Design review of the part built by this model. Coordinates are the model's own, in mm. A direction names the side the tool comes from. Give positions to 0.01 mm unless a question says otherwise; leave off trailing zeros. Order: outer loops, then holes, each group sorted by start corner. A loop starts at its lowest first (then second) coordinate and runs counter-clockwise, first axis right, second up. Notation, with made-up numbers: (-24, -34) -> (-6, -34) arc R15 cw to (-6, -17) -> close; hole circle Ø7 at (3, 52). An arc over 180 degrees is marked (long way). One line per item, written item: value. Start each with the question number.
1) Consider section B-B (z = 28). State the section outline as (x, y) points.
2) Consider section A-A (y = 101.5). State the section outline as (x, z) points.
3) Tool access review of faces 4 (the face through (-14.616, -3, 26)), 5 (the face through (16.42, -3.19, 45.49)), 6 (the face through (27, -3, 12.27)): name each direction out of +Z, -Z, +X, -X, +Y, -Y from which nothing blocks a thin tool from reaching the whole face with its end or side.
4) For pin 1 (9 mm diameter, centred on y = 33, z = 25, fed in from -X); pin 2 (1 mm diameter, centred on x = -26, y = 162.5, fed in from +Z); pin 3 (8 mm diameter, centred on x = -2.5, y = -14, fed in from +Z); pin 4 (12 mm diameter, centred on x = -29, z = 22.5, fed in from +Y), all flat-tipped, find the tip position at first contact; note any pin that passes through.
5) Wall thickness on line 1 along X through (y, z) = (58, 29); line 2 along Z through (x, y) = (34, 103.5); line 3 along Z through (x, y) = (18.5, -6): over which ranges is each line inside the solid? List them lowest first. Write a range as from..to.
6) The part is to be moulded in two halves that separate along Z. For faces 1 (the face through (1, -227.892, 19)), 2 (the face through (-26, -3, 12.27)), 3 (the face through (0.066, 3.19, 45.438)), say which applies: released by +Z, released by -Z, zero draft, split by the parting line, or undercut.
from build123d import *

# Parameters (mm, degrees)
F1_DEPTH    = 227.8918027878
F3_D        = 12.7
F4_T1_DEPTH = 455.7836055756
F4_T3_DEPTH = 473.2454690546
F4_T5_DEPTH = 481.1836055756
F4_T7_DEPTH = 475.2289422773


# Not quite as in the source:
# - a fillet or chamfer that OpenCascade refuses, or shapes differently, is made with other operations: its cross-section is extruded or revolved along the edge and cut away or added


with BuildPart() as f1:
    # F0 (on Front) → F1 (new body, symmetric)
    with BuildSketch(Plane.XZ):
        Polygon((-38.2542312145, 0), (0, 0), (38.2542312145, 0), (38.2542312145, 12.2701972723), (14.6159976721, 12.2701972723), (14.6159976721, 35.1866483688), (26.3448953629, 35.1866483688), (26.3448953629, 41.6826456785), (0, 51.7875403166), (-26.3448953629, 41.6826456785), (-26.3448953629, 35.1866483688), (-14.6159976721, 35.1866483688), (-14.6159976721, 12.2701972723), (-38.2542312145, 12.2701972723), align=None)
    extrude(amount=F1_DEPTH, both=True)

    # F3 (through all)
    with Locations(Plane.XZ.offset(227.8918027878)):
        with Locations((0, 51.7875403166)):
            Hole(F3_D / 2)

    # F4: fillet of radius 5.08 on 12 edges, made by hand

    # F4_s2 → F4_t1 (join)
    with BuildSketch(Plane.XZ.offset(-227.8918027878)):
        with BuildLine():
            ThreePointArc((-19.6959976721, 12.2701972723), (-16.1038952237, 13.7580948239), (-14.6159976721, 17.3501972723))
            Line((-14.6159976721, 17.3501972723), (-14.6159976721, 12.2701972723))
            Line((-14.6159976721, 12.2701972723), (-19.6959976721, 12.2701972723))
        make_face()
        with BuildLine():
            ThreePointArc((14.6159976721, 17.3501972723), (16.1038952237, 13.7580948239), (19.6959976721, 12.2701972723))
            Line((19.6959976721, 12.2701972723), (14.6159976721, 12.2701972723))
            Line((14.6159976721, 12.2701972723), (14.6159976721, 17.3501972723))
        make_face()
    extrude(amount=F4_T1_DEPTH)

    # F4_s4 → F4_t3 (cut)
    with BuildSketch(Plane.XZ.offset(-236.6227345273)):
        with BuildLine():
            ThreePointArc((23.0841549326, 42.9333410423), (25.4510773115, 41.0681681672), (26.3448953629, 38.1902729827))
            Line((26.3448953629, 38.1902729827), (26.3448953629, 41.6826456785))
            Line((26.3448953629, 41.6826456785), (23.0841549326, 42.9333410423))
        make_face()
        with BuildLine():
            ThreePointArc((-26.3448953629, 38.1902729827), (-25.4510773115, 41.0681681672), (-23.0841549326, 42.9333410423))
            Line((-23.0841549326, 42.9333410423), (-26.3448953629, 41.6826456785))
            Line((-26.3448953629, 41.6826456785), (-26.3448953629, 38.1902729827))
        make_face()
    extrude(amount=F4_T3_DEPTH, mode=Mode.SUBTRACT)

    # F4_s6 → F4_t5 (cut)
    with BuildSketch(Plane.XZ.offset(-240.5918027878)):
        with BuildLine():
            ThreePointArc((26.3448953629, 40.2666483688), (24.8569978113, 36.6745459204), (21.2648953629, 35.1866483688))
            Line((21.2648953629, 35.1866483688), (26.3448953629, 35.1866483688))
            Line((26.3448953629, 35.1866483688), (26.3448953629, 40.2666483688))
        make_face()
        with BuildLine():
            ThreePointArc((-21.2648953629, 35.1866483688), (-24.8569978113, 36.6745459204), (-26.3448953629, 40.2666483688))
            Line((-26.3448953629, 40.2666483688), (-26.3448953629, 35.1866483688))
            Line((-26.3448953629, 35.1866483688), (-21.2648953629, 35.1866483688))
        make_face()
        with BuildLine():
            ThreePointArc((38.2542312145, 7.1901972723), (36.766333663, 10.7822997207), (33.1742312145, 12.2701972723))
            Line((33.1742312145, 12.2701972723), (38.2542312145, 12.2701972723))
            Line((38.2542312145, 12.2701972723), (38.2542312145, 7.1901972723))
        make_face()
        with BuildLine():
            ThreePointArc((33.1742312145, 0), (36.766333663, 1.4878975516), (38.2542312145, 5.08))
            Line((38.2542312145, 5.08), (38.2542312145, 0))
            Line((38.2542312145, 0), (33.1742312145, 0))
        make_face()
        with BuildLine():
            ThreePointArc((-38.2542312145, 7.1901972723), (-36.766333663, 10.7822997207), (-33.1742312145, 12.2701972723))
            Line((-33.1742312145, 12.2701972723), (-38.2542312145, 12.2701972723))
            Line((-38.2542312145, 12.2701972723), (-38.2542312145, 7.1901972723))
        make_face()
        with BuildLine():
            ThreePointArc((-33.1742312145, 0), (-36.766333663, 1.4878975516), (-38.2542312145, 5.08))
            Line((-38.2542312145, 5.08), (-38.2542312145, 0))
            Line((-38.2542312145, 0), (-33.1742312145, 0))
        make_face()
    extrude(amount=F4_T5_DEPTH, mode=Mode.SUBTRACT)

    # F4_s8 → F4_t7 (cut)
    with BuildSketch(Plane.XZ.offset(-237.6144711386)):
        with BuildLine():
            ThreePointArc((-9.5599593035, 48.120705426), (-6.7869567139, 48.367304114), (-4.300388741, 47.1153720109))
            ThreePointArc((-4.300388741, 47.1153720109), (-5.2532816874, 48.2202540213), (-5.9288350745, 49.5134658544))
            Line((-5.9288350745, 49.5134658544), (-9.5599593035, 48.120705426))
        make_face()
        with BuildLine():
            ThreePointArc((4.300388741, 47.1153720109), (6.7869567139, 48.367304114), (9.5599593035, 48.120705426))
            Line((9.5599593035, 48.120705426), (5.9288350745, 49.5134658544))
            ThreePointArc((5.9288350745, 49.5134658544), (5.2532816874, 48.2202540213), (4.300388741, 47.1153720109))
        make_face()
    extrude(amount=F4_T7_DEPTH, mode=Mode.SUBTRACT)


solid = f1.part
Checked values:
1. outline: (-14.62, -227.89) -> (14.62, -227.89) -> (14.62, 227.89) -> (-14.62, 227.89) -> close
2. outline: (-38.25, 5.08) arc R5.08 ccw to (-33.17, 0) -> (33.17, 0) arc R5.08 ccw to (38.25, 5.08) -> (38.25, 7.19) arc R5.08 ccw to (33.17, 12.27) -> (19.7, 12.27) arc R5.08 cw to (14.62, 17.35) -> (14.62, 35.19) -> (21.26, 35.19) arc R5.08 ccw to (26.24, 39.23) arc R5.08 ccw to (23.08, 42.93) -> (9.56, 48.12) arc R5.08 ccw to (4.3, 47.12) arc R6.35 cw to (-4.3, 47.12) arc R5.08 ccw to (-9.56, 48.12) -> (-23.08, 42.93) arc R5.08 ccw to (-26.24, 39.23) arc R5.08 ccw to (-21.26, 35.19) -> (-14.62, 35.19) -> (-14.62, 17.35) arc R5.08 cw to (-19.7, 12.27) -> (-33.17, 12.27) arc R5.08 ccw to (-38.25, 7.19) -> close
3. face 4: -X, +Y, -Y
3. face 5: +Z, +X, +Y, -Y
3. face 6: +X, +Y, -Y
4. pin 1: stops at x = -14.62
4. pin 2: stops at z = 41
4. pin 3: stops at z = 48.3
4. pin 4: passes through
5. line 1: x = -14.62..14.62
5. line 2: z = 0.07..12.2
5. line 3: z = 0..12.41, 35.19..44.69
6. face 1: zero draft
6. face 2: undercut
6. face 3: released by +Z
